from build123d import *

# Parameters (mm, degrees)
F0_W     = 103.720352
F0_H     = 10.356933
F1_DEPTH = 4.796078
F2_R     = 8.331013
F3_DEPTH = 4.927844
F4_R     = 2.215122
F5_DEPTH = 5.888587


with BuildPart() as f1:
    # F0 (on Top) → F1 (new body)
    with BuildSketch(Plane.XY):
        with Locations((12.965046, 23.803338)):
            Rectangle(F0_W, F0_H)
    extrude(amount=F1_DEPTH)

    # F2 (on Top) → F3 (join)
    with BuildSketch(Plane.XY):
        with Locations((-41.580703, 24.02766)):
            Circle(F2_R)
    extrude(amount=F3_DEPTH)

    # F4 (on face) → F5 (join)
    with BuildSketch(Plane.XY.offset(4.927844)):
        with Locations((-41.580703, 24.02766)):
            Circle(F4_R)
    extrude(amount=F5_DEPTH)


solid = f1.part
Design review of the part built by this model. Coordinates are the model's own, in mm. A direction names the side the tool comes from. Round coordinates to 2 decimals unless told otherwise and drop trailing zeros. Loops run counter-clockwise (first coordinate to the right, second up) from the corner with the lowest first, then second, coordinate; pieces in that order, holes last. Notation, with made-up numbers: (-36, 21.5) - (11, 21.5) arc R19 ccw to (11, 49.5) - close; hole circle Ø7 at (-27.75, 65.5). An arc over 180 degrees is marked (long way). One line per item, written item: value. Start each with the question number.
1) To check wall thickness, follow L1, parallel to Z at x = 2, y = 23; L2, parallel to Y at x = -41.5, z = 9; L3, parallel to Z at x = -40, y = 21. State the ranges of each line that lie inside material, in increasing order. Write a range as from..to.
2) For faces 1 (the flat face through (14, 18.625, 2)), 2 (the cylindrical face through (-39.534, 23.179, 7.831)), 3 (the flat face through (14, 28.982, 2)), list the 3-axis set-ups (+Z, -Z, +X, -X, +Y, -Y) from which the entire face can be reached by the end or side of a thin tool; tool diameter is ignored.
3) Consider section A-A on z = 2.75. Give the boundary of the cut face in (x, y), then the cut area to 3 significant figures.
4) Insertion check: pin 1 Ø3 at (y, z) = (24, 7) entering from -X; pin 2 Ø4 at (x, z) = (2, 3) entering from -Y; pin 3 Ø4 at (x, z) = (-35.5, 4) entering from +Y. Each pin has a flat end and moves straight along its axis. Give the tip position at first contact, or say it passes through.
5) Consider section D-D on y = 20.5. Give the boundary of the cut face in (x, z).
6) Consider section C-C on y = 27.25. Give the boundary of the cut face in (x, z), then the cut area to 3 significant figures.
7) Consider section B-B on x = 44. Give the boundary of the cut face in (y, z).
Reported:
1. L1: z = 0..4.8
1. L2: y = 21.81..26.24
1. L3: z = 0..4.93
2. face 1: +Z, -Z, +X, -Y
2. face 2: +Z
2. face 3: +Z, -Z, +X, +Y
3. outline: (-35.24, 18.62) - (64.83, 18.62) - (64.83, 28.98) - (-34.88, 28.98) arc R8.33 ccw (long way) to start
3. area: 1,240 mm^2
4. pin 1: stops at x = -43.8
4. pin 2: stops at y = 18.62
4. pin 3: stops at y = 31.29
5. outline: (-49.13, 0) - (64.83, 0) - (64.83, 4.8) - (-34.03, 4.8) - (-34.03, 4.93) - (-49.13, 4.93) - close
6. outline: (-49.26, 0) - (64.83, 0) - (64.83, 4.8) - (-33.9, 4.8) - (-33.9, 4.93) - (-49.26, 4.93) - close
6. area: 549 mm^2
7. outline: (18.62, 0) - (28.98, 0) - (28.98, 4.8) - (18.62, 4.8) - close
